from build123d import *

# Parameters (mm, degrees)
SKETCH_1_W          = 6
SKETCH_1_H          = 6
EXTRUDE_1_DEPTH     = 30
CUT_EXTRUDE_1_REACH = 32.741
SKETCH_2_R          = 1.5
CUT_EXTRUDE_2_REACH = 32.741
SKETCH_3_R          = 1.5
SKETCH_4_R          = 1.5
CUT_EXTRUDE_3_DEPTH = 5
CUT_EXTRUDE_START   = -5
SKETCH_5_R          = 1.5
CUT_EXTRUDE_4_DEPTH = 5


with BuildPart() as part:
    # 草图1 → 凸台-拉伸1 (new body)
    with BuildSketch(Plane(origin=(0, 0, 0), x_dir=(1, 0, 0), z_dir=(0, 1, 0))):
        Rectangle(SKETCH_1_W, SKETCH_1_H)
    extrude(amount=EXTRUDE_1_DEPTH)

    # 草图2 → 切除-拉伸1 (cut, up to next)
    with BuildSketch(Plane.XY.offset(3), mode=Mode.PRIVATE) as cut_extrude_1_sk1:
        with Locations((0, 17.5)):
            Circle(SKETCH_2_R)
    cut_extrude_1_tool1 = extrude(cut_extrude_1_sk1.sketch, amount=-CUT_EXTRUDE_1_REACH, mode=Mode.PRIVATE) & part.part
    # 草图2 → 切除-拉伸1 (cut, up to next)
    with BuildSketch(Plane.XY.offset(3), mode=Mode.PRIVATE) as cut_extrude_1_sk2:
        with Locations((0, 7.5)):
            Circle(SKETCH_2_R)
    cut_extrude_1_tool2 = extrude(cut_extrude_1_sk2.sketch, amount=-CUT_EXTRUDE_1_REACH, mode=Mode.PRIVATE) & part.part
    add(cut_extrude_1_tool1.solids().sort_by_distance((0, 17.5, 3))[0], mode=Mode.SUBTRACT)
    add(cut_extrude_1_tool2.solids().sort_by_distance((0, 7.5, 3))[0], mode=Mode.SUBTRACT)

    # 草图3 → 切除-拉伸2 (cut, up to next)
    with BuildSketch(Plane(origin=(3, 0, 0), x_dir=(0, 0, -1), z_dir=(1, 0, 0)), mode=Mode.PRIVATE) as cut_extrude_2_sk1:
        with Locations((0, 22.5)):
            Circle(SKETCH_3_R)
    cut_extrude_2_tool1 = extrude(cut_extrude_2_sk1.sketch, amount=-CUT_EXTRUDE_2_REACH, mode=Mode.PRIVATE) & part.part
    # 草图3 → 切除-拉伸2 (cut, up to next)
    with BuildSketch(Plane(origin=(3, 0, 0), x_dir=(0, 0, -1), z_dir=(1, 0, 0)), mode=Mode.PRIVATE) as cut_extrude_2_sk2:
        with Locations((0, 12.5)):
            Circle(SKETCH_3_R)
    cut_extrude_2_tool2 = extrude(cut_extrude_2_sk2.sketch, amount=-CUT_EXTRUDE_2_REACH, mode=Mode.PRIVATE) & part.part
    add(cut_extrude_2_tool1.solids().sort_by_distance((3, 22.5, 0))[0], mode=Mode.SUBTRACT)
    add(cut_extrude_2_tool2.solids().sort_by_distance((3, 12.5, 0))[0], mode=Mode.SUBTRACT)

    # 草图4 → 切除-拉伸3 (cut)
    with BuildSketch(Plane(origin=(0, 30, 0), x_dir=(1, 0, 0), z_dir=(0, 1, 0))):
        with Locations(Location((0, 0, 0), (0, 0, 270))):
            Circle(SKETCH_4_R)
    extrude(amount=-CUT_EXTRUDE_3_DEPTH, mode=Mode.SUBTRACT)

    # 草图5 → 切除-拉伸4 (cut)
    with BuildSketch(Plane.XZ.offset(CUT_EXTRUDE_START)):
        with Locations(Location((0, 0, 0), (0, 0, 90))):
            Circle(SKETCH_5_R)
    extrude(amount=CUT_EXTRUDE_4_DEPTH, mode=Mode.SUBTRACT)


solid = part.part
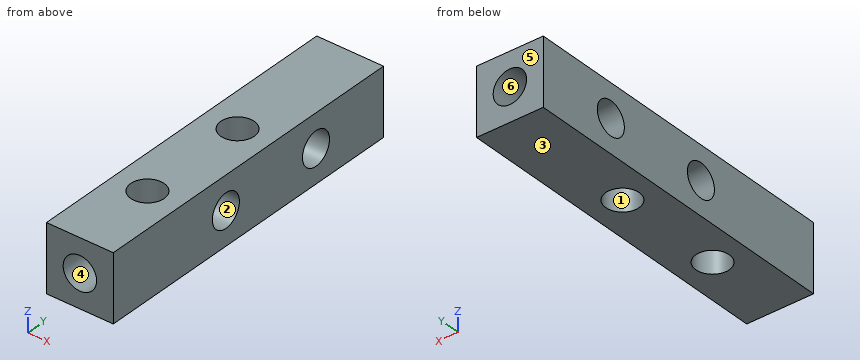
Check sheet for the modelled part. Datum: model origin and axes. Units: mm. Face numbers are marked on the shaded views. A direction names the side the tool comes from. Round coordinates to 2 decimals unless told otherwise and drop trailing zeros. Order: outer loops, then holes, each group sorted by start corner. A loop starts at its lowest first (then second) coordinate and runs counter-clockwise, first axis right, second up.
Q1. Depth check by flat-ended pin: P1, Ø2.5, axis at x = 0, z = 0, coming from the -Y side; P2, Ø2.5, axis at y = 12.5, z = 0, coming from the +X side. Enter the tip coordinate at first touch or a pass-through.
Filled sheet:
P1: stops at y = 5
P2: passes through
Q2. Scan lines: L1, parallel to X at y = 27.75, z = -0.05; L2, parallel to Y at x = -1.35, z = -2.7; L3, parallel to Y at x = -0.55, z = 2. Record each from-to range of solid material in increasing order.
Filled sheet:
L1: x = -3 to -1.5, 1.5 to 3
L2: y = 0 to 6.85, 8.15 to 16.85, 18.15 to 30
L3: y = 0 to 6.1, 8.9 to 16.1, 18.9 to 30
Q3. Cross-section at C-C, the plane z = 0. Enter the section's corners in (x, y).
Filled sheet:
outline: (-3, 0) - (-1.5, 0) - (-1.5, 5) - (1.5, 5) - (1.5, 0) - (3, 0) - (3, 11) - (-3, 11) - close; (-3, 14) - (3, 14) - (3, 21) - (-3, 21) - close; (-3, 24) - (3, 24) - (3, 30) - (1.5, 30) - (1.5, 25) - (-1.5, 25) - (-1.5, 30) - (-3, 30) - close; hole circle Ø3 at (0, 7.5); hole circle Ø3 at (0, 17.5)
Q4. Cross-section at A-A, the plane x = 0. Enter the section's corners in (y, z), plus the area to 3 significant figures.
Filled sheet:
outline: (0, -3) - (6, -3) - (6, 3) - (0, 3) - (0, 1.5) - (5, 1.5) - (5, -1.5) - (0, -1.5) - close; (9, -3) - (16, -3) - (16, 3) - (9, 3) - close; (19, -3) - (30, -3) - (30, -1.5) - (25, -1.5) - (25, 1.5) - (30, 1.5) - (30, 3) - (19, 3) - close; hole circle Ø3 at (12.5, 0); hole circle Ø3 at (22.5, 0)
area: 99.9 mm2
Q5. Set-up check for the marked faces 4, 5 and 6: record each of +Z, -Z, +X, -X, +Y, -Y from which the full face is reachable in a straight line by a thin tool's end or side.
Filled sheet:
face 4: -Y
face 5: +Z, -Z, +X, -X, +Y
face 6: +Y
Q6. Draft check along Z on the marked faces 1, 2 and 3. Enter one of: pulls with the +Z half, pulls with the -Z half, needs draft (parallel to the pull), parting line crosses it, or undercut.
Filled sheet:
face 1: needs draft
face 2: undercut
face 3: pulls with the -Z half
Q7. Cross-section at B-B, the plane y = 12.5. Enter the section's corners in (x, z).
Filled sheet:
outline: (-3, -3) - (3, -3) - (3, -1.5) - (-3, -1.5) - close; (-3, 1.5) - (3, 1.5) - (3, 3) - (-3, 3) - close
Q8. Cross-section at D-D, the plane x = -2.15. Enter the section's corners in (y, z), plus the area to 3 significant figures.
Filled sheet:
outline: (0, -3) - (30, -3) - (30, 3) - (0, 3) - close; hole circle Ø3 at (12.5, 0); hole circle Ø3 at (22.5, 0)
area: 166 mm2
